The drawing under review shows one solid part. Ordinate dimensions are in mm from its lowest x, y, z. A direction names the side the tool comes from. Round coordinates to 2 decimals unless told otherwise and drop trailing zeros. Order: outer loops, then holes, each group sorted by start corner. A loop starts at its lowest first (then second) coordinate and runs counter-clockwise, first axis right, second up. Notation, with made-up numbers: M -38.5,-26 L 12.5,-26 A18 ccw 12.5,4 Z; hole C 69,-21.75 d11. An arc over 180 degrees is marked long. Use a Markdown table: item, result.
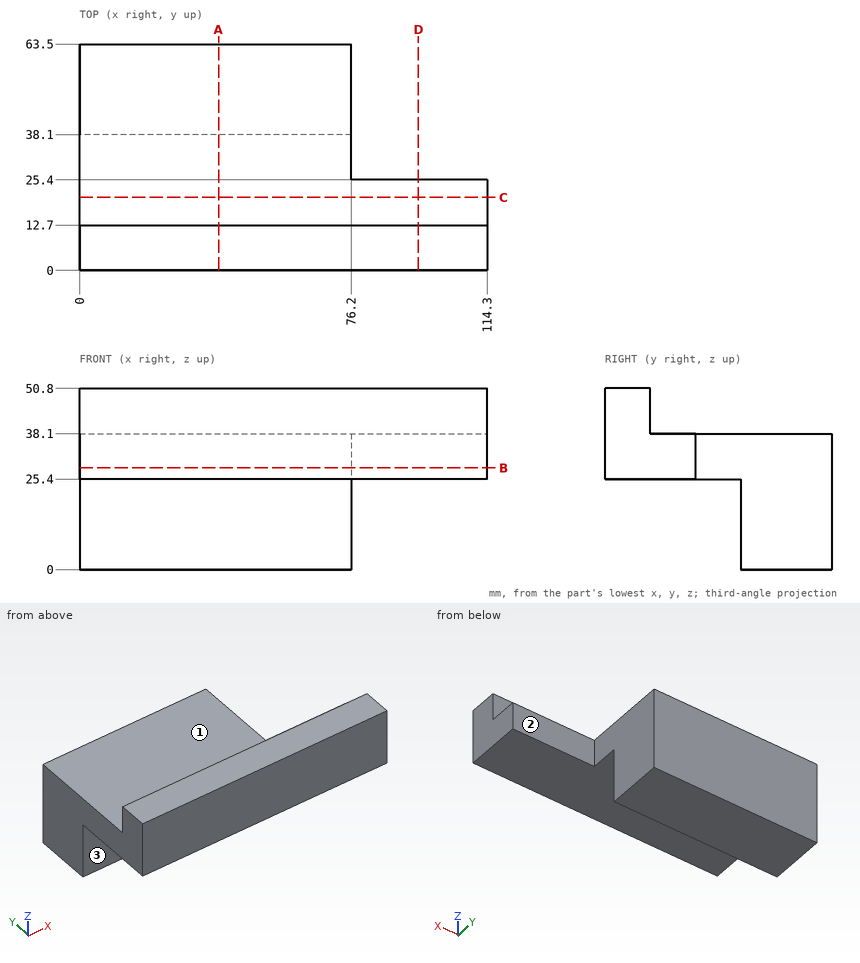
Q1. Add section D-D (x = 95). Write out the cut boundary in (y, z).
Determined:
| item | result |
|---|---|
| outline | M 0,25.4 L 25.4,25.4 L 25.4,38.1 L 12.7,38.1 L 12.7,50.8 L 0,50.8 Z |
Q2. Add section A-A (x = 39). Write out the cut boundary in (y, z).
Determined:
| item | result |
|---|---|
| outline | M 0,25.4 L 38.1,25.4 L 38.1,0 L 63.5,0 L 63.5,38.1 L 12.7,38.1 L 12.7,50.8 L 0,50.8 Z |
Q3. Add section C-C (y = 20.5). Write out the cut boundary in (x, z).
Determined:
| item | result |
|---|---|
| outline | M 0,25.4 L 114.3,25.4 L 114.3,38.1 L 0,38.1 Z |
Q4. Machinability: for the marked faces 1, 2 and 3, which of the approach directions +Z, -Z, +X, -X, +Y, -Y give a long, thin tool a straight path to every point of the face, cutting with its end or side? Answer none if there is none.
Determined:
| item | result |
|---|---|
| face 1 | +Z, +X, -X, +Y |
| face 2 | +Z, -Z, +X, +Y |
| face 3 | -Z, +X, -X, -Y |
Q5. Add section B-B (z = 28.5). Write out the cut boundary in (x, y).
Determined:
| item | result |
|---|---|
| outline | M 0,0 L 114.3,0 L 114.3,25.4 L 76.2,25.4 L 76.2,63.5 L 0,63.5 Z |
Q6. Wall thickness on line 1 along X through (y, z) = (46, 5); line 2 along Y through (x, z) = (107.5, 37.5); line 3 along Y through (x, z) = (18, 11): over which ranges is each line inside the solid? List them lowest first. Write a range as [from, to].
Determined:
| item | result |
|---|---|
| line 1 | x = [0, 76.2] |
| line 2 | y = [0, 25.4] |
| line 3 | y = [38.1, 63.5] |
Q7. Clearance check with flat-ended pins moving along their axes: pin 1 (1.5 mm diameter, centred on x = 54.5, y = 41.5, fed in from +Z); pin 2 (6.5 mm diameter, centred on x = 74, z = 47, fed in from +Y); pin 3 (4 mm diameter, centred on y = 55.5, z = 38, fed in from +X). State where each tip first meets the part, or that it passes through.
Determined:
| item | result |
|---|---|
| pin 1 | stops at z = 38.1 |
| pin 2 | stops at y = 12.7 |
| pin 3 | stops at x = 76.2 |
